Here's how the part is built. I have some questions about the finished solid (model axes, mm). A direction names the side the tool comes from. Give positions to 0.01 mm unless a question says otherwise; leave off trailing zeros. Loops run counter-clockwise (first coordinate to the right, second up) from the corner with the lowest first, then second, coordinate; pieces in that order, holes last.
Q1. Will these pins go through, and if not, where does the flat tip stop? P1, Ø1.8, axis at x = 14.88, y = -2.5, coming from the -Z side; P2, Ø4, axis at y = -79.5, z = -2.5, coming from the +X side; P3, Ø1.5, axis at x = 6, z = -11, coming from the +Y side; P4, Ø1.5, axis at x = -1.5, y = -27, coming from the -Z side.
Q2. If we section it at B-B (y = -2.5): Give the number of separate pieces and of enclosed holes in the cut face, plus the area to 3 significant figures.
Q3. For faces 4 (the face through (4.434, -2.465, 12.029)), 5 (the face through (2.545, -2.465, 12.688)), 6 (the face through (-11, -5, -8)), which set-ups out of +Z, -Z, +X, -X, +Y, -Y let a thin tool reach every point of the face, with its end or its side?
Q4. If we section it at A-A (y = -30): Please give me the cut outline in (x, z).
Q5. We'd pull the mould along Y, two halves only. Please class faces 1 (the face through (-14, 0, 9)), 2 (the face through (-1.2, -116.97, 12.81)), 3 (the face through (5.4, -2.46, -11.76)): +Y half, -Y half, draft (parallel to the pull), parting line (faces both ways), or undercut.
Q6. I need wall thicknesses on line 1 (Y direction, x = 3, z = -10); line 2 (X direction, y = -2.5, z = 0.65); line 3 (Y direction, x = 10, z = 11). Which ranges of each line are inside material? Lowest first, please.
from build123d import *

# Parameters (mm, degrees)
ESQUISSE1_R               = 10
BASE_DEPTH                = 120
BOSS_BALEINE_DEPTH        = 5
VIDE_BALEINE_DEPTH        = 3
REP_SUPPORT_BALEINE_COUNT = 5
CONGE_BALEINE_R           = 0.2
BOSS_EXTRU_3_START        = -5
BOSS_EXTRU_3_DEPTH        = 5
ENL_V_MAT_EXTRU_1_DEPTH   = 2
CONG_1_R                  = 0.2
CONG_1_OF_SYM_VIDE_BLOC_R = 0.2


with BuildPart() as part:
    # Esquisse1 → BASE (new body)
    with BuildSketch(Plane(origin=(0, 0, 0), x_dir=(1, 0, 0), z_dir=(0, 1, 0))):
        with Locations(Location((0, 0, 0), (0, 0, 270))):
            Circle(ESQUISSE1_R)
    extrude(amount=-BASE_DEPTH)

    # Esquisse2 → BOSS - BALEINE (add)
    with BuildSketch(Plane(origin=(0, 0, 0), x_dir=(1, 0, 0), z_dir=(0, 1, 0))):
        with BuildLine():
            ThreePointArc((9.38083152, -1.5), (9.486684928, -0.502801231), (9.486832981, 0.5))
            Line((9.486832981, 0.5), (17.38083152, 0.5))
            Line((17.38083152, 0.5), (17.38083152, -1.5))
            Line((17.38083152, -1.5), (9.38083152, -1.5))
        make_face()
    boss_baleine = extrude(amount=-BOSS_BALEINE_DEPTH)

    # Esquisse3 → VIDE - BALEINE (cut)
    with BuildSketch(Plane.XY.offset(1.5)):
        with BuildLine():
            Line((13.88083152, 0), (13.820171348, -1.439339828))
            ThreePointArc((13.820171348, -1.439339828), (14.88083152, -4), (15.941491691, -1.439339828))
            Line((15.941491691, -1.439339828), (15.88083152, 0))
            Line((15.88083152, 0), (13.88083152, 0))
        make_face()
    vide_baleine = extrude(amount=-VIDE_BALEINE_DEPTH, mode=Mode.SUBTRACT)

    # REP - SUPPORT BALEINE: BOSS - BALEINE, VIDE - BALEINE ×5 about axis
    rep_support_baleine_axis = Axis((0, 0, 0), (0, 1, 0))
    add([boss_baleine.rotate(rep_support_baleine_axis, i * 360 / REP_SUPPORT_BALEINE_COUNT) for i in range(1, REP_SUPPORT_BALEINE_COUNT)])
    add([vide_baleine.rotate(rep_support_baleine_axis, i * 360 / REP_SUPPORT_BALEINE_COUNT) for i in range(1, REP_SUPPORT_BALEINE_COUNT)], mode=Mode.SUBTRACT)

    # CONGE BALEINE
    conge_baleine_edges = [part.edges().sort_by_distance(p)[0] for p in [
        (4.764941094, 0, -13.046946771),
        (5.382975083, 0, -14.949059804),
        (-10.935935969, 0, -8.563456554),
        (-12.553969958, 0, -9.739027059),
        (-11.523721222, 0, 7.75443956),
        (-13.14175521, 0, 8.930010064),
        (3.813884577, 0, 13.355963766),
        (4.431918566, 0, 15.258076798),
        (13.88083152, 0, 0.5),
        (15.88083152, 0, 0.5),
    ]]
    fillet(conge_baleine_edges, radius=CONGE_BALEINE_R)

    # Esquisse4 → Boss.-Extru.3 (add)
    with BuildSketch(Plane.XZ.offset(120).offset(BOSS_EXTRU_3_START)):
        with BuildLine():
            ThreePointArc((10, 0), (-5.017525477, -8.650112027), (-4.964887617, 8.680431496))
            Line((-4.964887617, 8.680431496), (-6.781900496, 13.379305874))
            ThreePointArc((-6.781900496, 13.379305874), (5.409975206, -13.990431311), (-3.983814234, 14.461300915))
            Line((-3.983814234, 14.461300915), (-2.166801355, 9.762426537))
            ThreePointArc((-2.166801355, 9.762426537), (6.258273981, 7.799615809), (10, 0))
        make_face()
    extrude(amount=BOSS_EXTRU_3_DEPTH)

    # Esquisse5 → Enlèv. mat.-Extru.1 (cut)
    with BuildSketch(Plane(origin=(-1.399043131, 0, -0.540997521), x_dir=(0.36066501374715604, 0, -0.9326954207343167), z_dir=(0.9326954207343167, 0, 0.36066501374715604))):
        with BuildLine():
            Line((-13.470498479, -116.443357535), (-13.155835762, -115))
            Line((-13.155835762, -115), (-11.655835762, -115))
            Line((-11.655835762, -115), (-11.341173044, -116.443357535))
            ThreePointArc((-11.341173044, -116.443357535), (-12.405835762, -119), (-13.470498479, -116.443357535))
        make_face()
    enl_v_mat_extru_1 = extrude(amount=-ENL_V_MAT_EXTRU_1_DEPTH, mode=Mode.SUBTRACT)

    # Congé1
    cong_1_edges = [part.edges().sort_by_distance(p)[0] for p in [
        (-7.076588238, -115, 11.368725236),
        (-6.535590717, -115, 9.969682105),
    ]]
    fillet(cong_1_edges, radius=CONG_1_R)

    # SYM VIDE BLOC: Enlèv. mat.-Extru.1 across plane
    add(enl_v_mat_extru_1.mirror(Plane(origin=(0, 0, 0), x_dir=(-0.3606650137471561, 0, 0.9326954207343165), z_dir=(0.9326954207343167, 0, 0.36066501374715604))), mode=Mode.SUBTRACT)

    # Congé1 of SYM VIDE BLOC
    cong_1_of_sym_vide_bloc_edges = [part.edges().sort_by_distance(p)[0] for p in [
        (-2.413111134, -115, 13.172050305),
        (-1.872113613, -115, 11.773007174),
    ]]
    fillet(cong_1_of_sym_vide_bloc_edges, radius=CONG_1_OF_SYM_VIDE_BLOC_R)


solid = part.part
Check sheet entries:
1. P1: passes through
1. P2: stops at x = 9.99
1. P3: stops at y = -115
1. P4: stops at z = -9.97
2. separate pieces: 6
2. enclosed holes: 0
2. area: 358 mm2
3. face 4: +X, +Y
3. face 5: +Z, +Y
3. face 6: -Z, -X
4. outline: circle Ø20 at (0, 0)
5. face 1: +Y half
5. face 2: undercut
5. face 3: draft
6. line 1: y = -120 to -115, -5 to 0
6. line 2: x = -9.98 to 13.38, 16.38 to 17.38
6. line 3: y = -120 to -115
